Verification items for the finished model (mm, model axes). A direction names the side the tool comes from. Round coordinates to 2 decimals unless told otherwise and drop trailing zeros. Write each loop counter-clockwise with the first axis right and the second up, starting at its lowest first coordinate (ties: lowest second). Pieces come first, ordered by that corner, then holes. Notation, with made-up numbers: M 46,25.25 L 68,25.25 A17 ccw 68,32.25 Z; hole C 9,7 d1. An arc over 180 degrees is marked long. Answer in a Markdown table with one row per item. Add a question column.
1. Draft check along Z on faces 5 (the cylindrical face through (-18.996, 7.786, 85.546)), 6 (the cylindrical face through (74.96, 7.51, 47.79)), 7 (the flat face through (-19, 0, -1)). Enter one of: pulls with the +Z half, pulls with the -Z half, needs draft (parallel to the pull), parting line crosses it, or undercut.
2. Go/stop test with flat-tipped pins: pin 1 Ø12 at (y, z) = (7.5, -44) entering from +X; pin 2 Ø10 at (x, y) = (59.5, 12) entering from +Z; pin 3 Ø3 at (x, z) = (-32.07, -55.54) entering from -Y. Record where each tip stops, or that it passes through.
3. Sectioned sample at B-B on y = 5.5. Record the cut outline in (x, z) (3 decimals).
4. Material ranges on probe 1 along X at (y, z) = (7, -5.5); probe 2 along Y at (x, z) = (1, -26.5); probe 3 along Z at (x, y) = (-50, 6), recorded low to high.
5. Set-up check for faces 1 (the cylindrical face through (7.7, -6.3, -10.1)), 2 (the conical face through (40.82, 19.87, -12.85)), 3 (the flat face through (-7, 15.24, 7)), 4 (the flat face through (0, -12.7, 0)): record each of +Z, -Z, +X, -X, +Y, -Y from which the full face is reachable in a straight line by a thin tool's end or side.
```python
from build123d import *

# Parameters (mm, degrees)
SKETCH1_R           = 88.9
BOSS_EXTRUDE1_DEPTH = 15.24
SKETCH2_R           = 39.37
BOSS_EXTRUDE2_DEPTH = 6.35
SKETCH4_R           = 39.37
CUT_EXTRUDE1_DEPTH  = 6.35
FILLET1_R           = 6.35
SKETCH5_R           = 9.525
CUT_EXTRUDE2_DEPTH  = 12.7
SKETCH8_R           = 1.27
CUT_EXTRUDE3_DEPTH  = 6.35
CIRPATTERN1_COUNT   = 6
SKETCH9_R           = 12.7
BOSS_EXTRUDE3_DEPTH = 12.7


# Read off the part's stored shape, not the designer's step: Shell1
with BuildPart() as part:
    # Sketch1 → Boss-Extrude1 (new body)
    with BuildSketch(Plane(origin=(0, 0, 0), x_dir=(1, 0, 0), z_dir=(0, 1, 0))):
        with Locations(Location((0, 0, 0), (0, 0, 270))):
            Circle(SKETCH1_R)
    extrude(amount=BOSS_EXTRUDE1_DEPTH)

    # Sketch2 → Boss-Extrude2 (add)
    with BuildSketch(Plane(origin=(0, 15.24, 0), x_dir=(1, 0, 0), z_dir=(0, 1, 0))):
        with Locations(Location((0, 0, 0), (0, 0, 270))):
            Circle(SKETCH2_R)
    extrude(amount=BOSS_EXTRUDE2_DEPTH)

    # Sketch3 → Revolve1 (revolve)
    with BuildSketch(Plane(origin=(0, 0, 0), x_dir=(0, 0, -1), z_dir=(1, 0, 0)), mode=Mode.PRIVATE) as revolve1_sk:
        Polygon((-39.37, 21.59), (-39.37, 15.24), (-88.9, 15.24), align=None)
    revolve(revolve1_sk.sketch.rotate(Axis((0, 0, 0), (0, 1, 0)), 180), axis=Axis((0, 0, 0), (0, 1, 0)))

    # Sketch4 → Cut-Extrude1 (cut)
    with BuildSketch(Plane(origin=(0, 21.59, 0), x_dir=(1, 0, 0), z_dir=(0, 1, 0))):
        with Locations(Location((0, 0, 0), (0, 0, 270))):
            Circle(SKETCH4_R)
    extrude(amount=-CUT_EXTRUDE1_DEPTH, mode=Mode.SUBTRACT)

    # Fillet1
    fillet1_edges = [part.edges().sort_by_distance(p)[0] for p in [
        (0, 15.24, -39.37),
    ]]
    fillet(fillet1_edges, radius=FILLET1_R - 0.0001)  # a hair under: the kernel refuses the full size

    # Sketch5 → Cut-Extrude2 (cut)
    with BuildSketch(Plane(origin=(0, 15.24, 0), x_dir=(1, 0, 0), z_dir=(0, 1, 0))):
        with Locations(Location((0, 0, 0), (0, 0, 270))):
            Circle(SKETCH5_R)
    extrude(amount=-CUT_EXTRUDE2_DEPTH, mode=Mode.SUBTRACT)

    # Shell1 outline → Shell1 (revolve, cut)
    with BuildSketch(Plane.XY):
        with BuildLine():
            Line((87.63, 14.12242584), (40.505388812, 20.164042659))
            ThreePointArc((40.505388812, 20.164042659), (37.877911334, 15.71930179), (33.02, 13.97))
            Line((33.02, 13.97), (10.795, 13.97))
            Line((10.795, 13.97), (10.795, 2.54))
            Line((10.795, 2.54), (0, 2.54))
            Line((0, 2.54), (0, 1.27))
            Line((0, 1.27), (87.63, 1.27))
            Line((87.63, 1.27), (87.63, 14.12242584))
        make_face()
    revolve(axis=Axis((0, 0, 0), (0, 1, 0)), mode=Mode.SUBTRACT)

    # Sketch8 → Cut-Extrude3 (cut)
    with BuildSketch(Plane(origin=(0, 15.24, 0), x_dir=(-1, 0, 0), z_dir=(0, -1, 0))):
        with Locations(Location((-64.135, 0, 0), (0, 0, 65.776295288))):
            Circle(SKETCH8_R)
    cut_extrude3 = extrude(amount=-CUT_EXTRUDE3_DEPTH, mode=Mode.SUBTRACT)

    # CirPattern1: Cut-Extrude3 ×6 about axis
    cirpattern1_axis = Axis((0, 0, 0), (0, 1, 0))
    for i in range(1, CIRPATTERN1_COUNT):
        add(cut_extrude3.rotate(cirpattern1_axis, i * 360 / CIRPATTERN1_COUNT), mode=Mode.SUBTRACT)

    # Sketch9 → Boss-Extrude3 (add)
    with BuildSketch(Plane.XZ):
        with Locations(Location((0, 0, 0), (0, 0, 90))):
            Circle(SKETCH9_R)
    extrude(amount=BOSS_EXTRUDE3_DEPTH)


solid = part.part
```
Geometry check:
| question | item | result |
|---|---|---|
| 1 | face 5 | undercut |
| 1 | face 6 | parting line crosses it |
| 1 | face 7 | needs draft |
| 2 | pin 1 | stops at x = 80.37 |
| 2 | pin 2 | stops at z = 70.24 |
| 2 | pin 3 | stops at y = 0 |
| 3 | outline | C 0,0 d177.8; C 0,0 d21.59; hole C 0,0 d175.26; hole C 0,0 d19.05 |
| 4 | probe 1 | x = -88.73 to -87.46, -9.29 to -7.78, 7.78 to 9.29, 87.46 to 88.73 |
| 4 | probe 2 | y = 0 to 1.27, 13.97 to 15.24 |
| 4 | probe 3 | z = -73.51 to -71.97, 71.97 to 73.51 |
| 5 | face 1 | -Y |
| 5 | face 2 | none |
| 5 | face 3 | +Y |
| 5 | face 4 | +Z, -Z, +X, -X, -Y |
